Model file for the job. Use its own axes, mm. A direction names the side the tool comes from. Give positions to 0.01 mm unless a question says otherwise; leave off trailing zeros. Write each loop counter-clockwise with the first axis right and the second up, starting at its lowest first coordinate (ties: lowest second). Pieces come first, ordered by that corner, then holes.
```python
from build123d import *

# Parameters (mm, degrees)
SKETCH1_R           = 3.75
BOSS_EXTRUDE1_DEPTH = 23.75
SKETCH2_W           = 30
SKETCH2_H           = 47.5
BOSS_EXTRUDE2_DEPTH = 5
SKETCH3_W           = 37.5
SKETCH3_H           = 21.575563825
CUT_EXTRUDE1_DEPTH  = 30
SKETCH4_R           = 1.5
CUT_EXTRUDE2_DEPTH  = 5


with BuildPart() as part:
    # Sketch1 → Boss-Extrude1 (new body, symmetric)
    with BuildSketch(Plane.XY):
        with BuildLine():
            Line((-15, -10), (15, -10))
            Line((15, -10), (9.230769231, 3.846153846))
            ThreePointArc((9.230769231, 3.846153846), (0, 10), (-9.230769231, 3.846153846))
            Line((-9.230769231, 3.846153846), (-15, -10))
        make_face()
        Circle(SKETCH1_R, mode=Mode.SUBTRACT)
    extrude(amount=BOSS_EXTRUDE1_DEPTH, both=True)

    # Sketch2 → Boss-Extrude2 (add)
    with BuildSketch(Plane.XZ.offset(10)):
        Rectangle(SKETCH2_W, SKETCH2_H)
    extrude(amount=BOSS_EXTRUDE2_DEPTH)

    # Sketch3 → Cut-Extrude1 (cut)
    with BuildSketch(Plane(origin=(15, 0, 0), x_dir=(0, 0, -1), z_dir=(1, 0, 0))):
        with Locations((0, 0.787781913)):
            Rectangle(SKETCH3_W, SKETCH3_H)
    extrude(amount=-CUT_EXTRUDE1_DEPTH, mode=Mode.SUBTRACT)

    # Sketch4 → Cut-Extrude2 (cut)
    with BuildSketch(Plane(origin=(0, -10, 0), x_dir=(1, 0, 0), z_dir=(0, 1, 0))):
        with Locations((-10, 13.75)):
            Circle(SKETCH4_R)
        with Locations((10, -13.75)):
            Circle(SKETCH4_R)
        with Locations((-10, -13.75)):
            Circle(SKETCH4_R)
        with Locations((10, 13.75)):
            Circle(SKETCH4_R)
    extrude(amount=-CUT_EXTRUDE2_DEPTH, mode=Mode.SUBTRACT)


solid = part.part
```
1. Slice it at A-A, the plane x = 0. Write the cut outline in (y, z).
Calculated:
outline: (-15, -23.75) - (-3.75, -23.75) - (-3.75, -18.75) - (-10, -18.75) - (-10, 18.75) - (-3.75, 18.75) - (-3.75, 23.75) - (-15, 23.75) - close; (3.75, -23.75) - (10, -23.75) - (10, -18.75) - (3.75, -18.75) - close; (3.75, 18.75) - (10, 18.75) - (10, 23.75) - (3.75, 23.75) - close
2. Probe probe 1 along X at (y, z) = (-13.65, 13.75); probe 2 along Z at (x, y) = (10, -13.25); probe 3 along Z at (x, y) = (7.5, 4). List the from-to ranges inside material, lowest first.
Calculated:
probe 1: x = -15 to -11.5, -8.5 to 8.5, 11.5 to 15
probe 2: z = -23.75 to -15.25, -12.25 to 12.25, 15.25 to 23.75
probe 3: z = -23.75 to -18.75, 18.75 to 23.75
3. Pull direction X, two halves, no side cores. Call faces 3 (the flat face through (0, -15, 0)), 4 (the flat face through (-15, -12, 0)), 5 (the cylindrical face through (-11.5, -12.5, -13.8)): +X half, -X half, draft (parallel to the pull), parting line (faces both ways), or undercut.
Calculated:
face 3: draft
face 4: -X half
face 5: undercut
4. Slice it at D-D, the plane z = 13.75. Write the cut outline in (x, y).
Calculated:
outline: (-15, -15) - (-11.5, -15) - (-11.5, -10) - (-15, -10) - close; (-8.5, -15) - (8.5, -15) - (8.5, -10) - (-8.5, -10) - close; (11.5, -15) - (15, -15) - (15, -10) - (11.5, -10) - close
5. Pin check, flat tips, straight feed: P1, Ø1, axis at x = 7.5, z = 14, coming from the +Y side; P2, Ø4, axis at y = -7, z = 18.5, coming from the -X side. Stop position of each tip, or through.
Calculated:
P1: stops at y = -10
P2: stops at x = -14.58
6. Slice it at B-B, the plane z = -20. Write the cut outline in (x, y).
Calculated:
outline: (-15, -15) - (15, -15) - (15, -10) - (9.23, 3.85) arc R10 ccw to (-9.23, 3.85) - (-15, -10) - close; hole circle Ø7.5 at (0, 0)
7. Slice it at C-C, the plane y = 5.5. Write the cut outline in (x, z).
Calculated:
outline: (-8.35, -23.75) - (8.35, -23.75) - (8.35, -18.75) - (-8.35, -18.75) - close; (-8.35, 18.75) - (8.35, 18.75) - (8.35, 23.75) - (-8.35, 23.75) - close
8. Which spindle directions (+Z, -Z, +X, -X, +Y, -Y) get a long thin tool onto all of the face, cutting with end or side? Do faces 1 (the flat face through (0, -5, 18.75)), 2 (the flat face through (15, -12, 0)). Say none if no direction does.
Calculated:
face 1: +X, -X, +Y
face 2: +Z, -Z, +X, +Y, -Y
